The listing builds one solid part. Answer for the finished solid, in the listing's coordinates (mm). Coordinates: 2 decimals unless noted, no trailing zeros. Order: outer loops, then holes, each group sorted by start corner. A loop starts at its lowest first (then second) coordinate and runs counter-clockwise, first axis right, second up.
from build123d import *

# Parameters (mm, degrees)
SKETCH2_W           = 35
SKETCH2_H           = 25
BOSS_EXTRUDE1_DEPTH = 1.4
FILLET1_R           = 3
SKETCH3_R           = 5
CUT_EXTRUDE1_DEPTH  = 22.551334065


with BuildPart() as part:
    # Sketch2 → Boss-Extrude1 (new body)
    with BuildSketch(Plane(origin=(0, 0, 0), x_dir=(1, 0, 0), z_dir=(0, 1, 0))):
        Rectangle(SKETCH2_W, SKETCH2_H)
    extrude(amount=BOSS_EXTRUDE1_DEPTH)

    # Fillet1
    fillet1_edges = [part.edges().sort_by_distance(p)[0] for p in [
        (17.5, 0.7, 12.5),
        (-17.5, 0.7, 12.5),
        (-17.5, 0.7, -12.5),
        (17.5, 0.7, -12.5),
    ]]
    fillet(fillet1_edges, radius=FILLET1_R)

    # Sketch3 → Cut-Extrude1 (cut, through all)
    with BuildSketch(Plane(origin=(0, 1.4, 0), x_dir=(1, 0, 0), z_dir=(0, 1, 0))):
        with Locations(Location((0, 0, 0), (0, 0, 270))):
            Circle(SKETCH3_R)
    extrude(amount=-CUT_EXTRUDE1_DEPTH, mode=Mode.SUBTRACT)


solid = part.part
1) Section C-C (x = 0) is taken. Give the vertices of the cut face in (y, z), then the cut area to 3 significant figures.
2) Determine the mould class of faces 1 (the face through (-4.88, 0.71, -1.08)), 2 (the face through (0, 1.4, -6)), 3 (the face through (-16.64, 0.71, 11.6)) for opening direction Z: released by +Z, released by -Z, zero draft, split by the parting line, or undercut.
3) Consider L1, parallel to X at y = 0.95, z = 0; L2, parallel to Z at x = 3, y = 0.1; L3, parallel to X at y = 0.75, z = 2. Determine where each line is inside the solid, lowest interval first.
4) Section B-B (y = 0.45) is taken. Give the vertices of the cut face in (x, z).
5) Section A-A (z = 0) is taken. Give the vertices of the cut face in (x, y), then the cut area to 3 significant figures.
6) This flat-tipped pin is pushed along its axis until it touches: P1, Ø13, axis at x = 0, z = 0, coming from the +Y side. Where does it stop, or does it pass through?
Filled sheet:
1. outline: (0, -12.5) - (1.4, -12.5) - (1.4, -5) - (0, -5) - close; (0, 5) - (1.4, 5) - (1.4, 12.5) - (0, 12.5) - close
1. area: 21.0 mm2
2. face 1: undercut
2. face 2: zero draft
2. face 3: released by +Z
3. L1: x = -17.5 to -5, 5 to 17.5
3. L2: z = -12.5 to -4, 4 to 12.5
3. L3: x = -17.5 to -4.58, 4.58 to 17.5
4. outline: (-17.5, -9.5) arc R3 ccw to (-14.5, -12.5) - (14.5, -12.5) arc R3 ccw to (17.5, -9.5) - (17.5, 9.5) arc R3 ccw to (14.5, 12.5) - (-14.5, 12.5) arc R3 ccw to (-17.5, 9.5) - close; hole circle Ø10 at (0, 0)
5. outline: (-17.5, 0) - (-5, 0) - (-5, 1.4) - (-17.5, 1.4) - close; (5, 0) - (17.5, 0) - (17.5, 1.4) - (5, 1.4) - close
5. area: 35.0 mm2
6. P1: stops at y = 1.4
